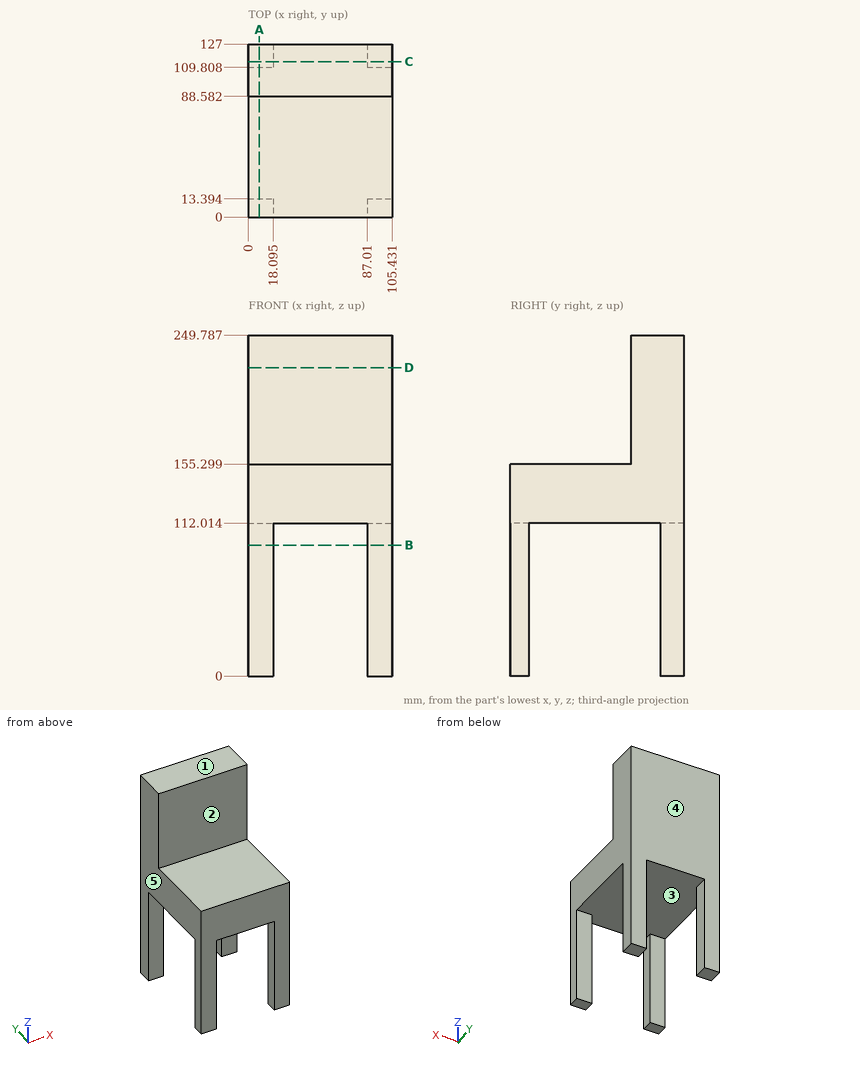
Could you check a few things on this drawing? It's one solid part, dimensions in mm from its lowest x, y, z. A direction names the side the tool comes from. Round coordinates to 2 decimals unless told otherwise and drop trailing zeros. Order: outer loops, then holes, each group sorted by start corner. A loop starts at its lowest first (then second) coordinate and runs counter-clockwise, first axis right, second up.
(1) If we mould it in two halves opening along X, with no side actions, what happens to the marked faces 3, 4 and 5? For each: released by +X, released by -X, zero draft, split by the parting line, or undercut.
Response values:
face 3: undercut
face 4: zero draft
face 5: released by -X
(2) Imagine slicing it at A-A (x = 8). Write out the boundary of the cut face in (y, z).
Response values:
outline: (0, 0) - (13.39, 0) - (13.39, 112.01) - (109.81, 112.01) - (109.81, 0) - (127, 0) - (127, 249.79) - (88.58, 249.79) - (88.58, 155.3) - (0, 155.3) - close
(3) I'm going to push a flat-ended pin straight in: pin 1 (3 mm diameter, centred on x = 31.5, y = 82, fed in from +Z). Where does the tip first touch, or does it pass through?
Response values:
pin 1: stops at z = 155.3
(4) Imagine slicing it at D-D (z = 226). Write out the boundary of the cut face in (x, y), plus the area to 3 significant figures.
Response values:
outline: (0, 88.58) - (105.43, 88.58) - (105.43, 127) - (0, 127) - close
area: 4,050 mm2
(5) Imagine slicing it at B-B (z = 96). Write out the boundary of the cut face in (x, y) (1 decimal), plus the area to 3 significant figures.
Response values:
outline: (0, 0) - (18.1, 0) - (18.1, 13.4) - (0, 13.4) - close; (0, 109.8) - (18.1, 109.8) - (18.1, 127) - (0, 127) - close; (87, 0) - (105.4, 0) - (105.4, 13.4) - (87, 13.4) - close; (87, 109.8) - (105.4, 109.8) - (105.4, 127) - (87, 127) - close
area: 1,120 mm2
(6) Please list where these lines run through material, in increasing order: line 1 along Y through (x, z) = (7.5, 31); line 2 along X through (y, z) = (116.5, 84) (1 decimal); line 3 along Y through (x, z) = (59.5, 170.5).
Response values:
line 1: y = 0 to 13.39, 109.81 to 127
line 2: x = 0 to 18.1, 87 to 105.4
line 3: y = 88.58 to 127
(7) Imagine slicing it at C-C (y = 114). Write out the boundary of the cut face in (x, z) (1 decimal), plus the area to 3 significant figures.
Response values:
outline: (0, 0) - (18.1, 0) - (18.1, 112) - (87, 112) - (87, 0) - (105.4, 0) - (105.4, 249.8) - (0, 249.8) - close
area: 18,600 mm2
(8) Which directions (+Z, -Z, +X, -X, +Y, -Y) give clear straight access to the entire face, cutting with the end or side of a thin tool? Please do the marked faces 1 and 2.
Response values:
face 1: +Z, +X, -X, +Y, -Y
face 2: +Z, +X, -X, -Y
